Could you check a few things on this model? Use its own coordinates, in mm. A direction names the side the tool comes from. Round coordinates to 2 decimals unless told otherwise and drop trailing zeros. Loops run counter-clockwise (first coordinate to the right, second up) from the corner with the lowest first, then second, coordinate; pieces in that order, holes last. Notation, with made-up numbers: (-30.75, 71.25) -> (-7.75, 71.25) arc R25 cw to (-7.75, 102.25) -> close; hole circle Ø10 at (83.5, 41). An arc over 180 degrees is marked (long way). Put each result on its own line as item: value. Start each with the question number.
1. I need wall thicknesses on line 1 (X direction, y = 0.5, z = 0.6); line 2 (Z direction, x = -34, y = -3.5); line 3 (Y direction, x = -61.5, z = -0.9). Which ranges of each line are inside material? Lowest first, please. Write a range as [from, to].
2. Imagine slicing it at A-A, the plane y = -9. Please give me the cut outline in (x, z), and give its area (3 significant figures).
3. Imagine slicing it at D-D, the plane x = -38.5. Please give me the cut outline in (y, z).
4. Imagine slicing it at C-C, the plane y = -0.5. Please give me the cut outline in (x, z), and give its area (3 significant figures).
5. If we mould it in two halves opening along X, with no side actions, what happens to faces 1 (the flat face through (-43.491, -9, 2)), 2 (the flat face through (-72.441, 13, 2)), 3 (the flat face through (-40, 0, -1.5))? For each: pulls with the +X half, pulls with the -X half, needs draft (parallel to the pull), parting line crosses it, or undercut.
6. Which directions (+Z, -Z, +X, -X, +Y, -Y) give clear straight access to the entire face, cutting with the end or side of a thin tool? Please do faces 4 (the flat face through (-48, 9, 2)), 5 (the flat face through (-60, 20, -1.5)), 6 (the cylindrical face through (-38.1, 17.54, -0.74)), 7 (the flat face through (-55.991, -9, 2)).
7. I'm going to push flat-ended pins straight in: P1, Ø8, axis at x = -49.74, y = 10.11, coming from the -Z side; P2, Ø1.8, axis at x = -49.5, y = 8.5, coming from the +Z side; P3, Ø1.6, axis at x = -48.5, z = 2.5, coming from the -Y side; P4, Ø4, axis at x = -47, y = -6.5, coming from the -Z side. Where does each tip first touch, or does it pass through?
8. Imagine slicing it at B-B, the plane x = -45.5. Please give me the cut outline in (y, z).
```python
from build123d import *

# Parameters (mm, degrees)
SKETCH_1_W          = 45.4
SKETCH_1_H          = 61
EXTRUDE_1_DEPTH     = 4
SKETCH_2_W          = 12.5
SKETCH_2_H          = 18
CUT_EXTRUDE_1_DEPTH = 3.2
SKETCH_4_R          = 1.6
CUT_EXTRUDE_2_DEPTH = 10
SKETCH_5_R          = 3
CUT_EXTRUDE_3_DEPTH = 2
SKETCH_3_R          = 3.05
EXTRUDE_2_DEPTH     = 1.5


with BuildPart() as part:
    # 草图1 → 凸台-拉伸1 (new body)
    with BuildSketch(Plane.XY):
        with Locations((-49.741035857, 13.111663348)):
            Rectangle(SKETCH_1_W, SKETCH_1_H)
    extrude(amount=EXTRUDE_1_DEPTH)

    # 草图2 → 切除-拉伸1 (cut)
    with BuildSketch(Plane(origin=(0, 0, 0), x_dir=(-1, 0, 0), z_dir=(0, 0, -1))):
        with Locations((49.741035857, -8.388336652)):
            Rectangle(SKETCH_2_W, SKETCH_2_H)
    extrude(amount=-CUT_EXTRUDE_1_DEPTH, mode=Mode.SUBTRACT)

    # 草图4 → 切除-拉伸2 (cut)
    with BuildSketch(Plane.XY.offset(4)):
        with Locations((-49.741035857, 10.111663348)):
            Circle(SKETCH_4_R)
    extrude(amount=-CUT_EXTRUDE_2_DEPTH, mode=Mode.SUBTRACT)

    # 草图5 → 切除-拉伸3 (cut)
    with BuildSketch(Plane.XY.offset(4)):
        with Locations((-49.741035857, 10.111663348)):
            Circle(SKETCH_5_R)
    extrude(amount=-CUT_EXTRUDE_3_DEPTH, mode=Mode.SUBTRACT)

    # 草图3 → 凸台-拉伸2 (add)
    with BuildSketch(Plane(origin=(0, 0, 0), x_dir=(-1, 0, 0), z_dir=(0, 0, -1))):
        with Locations(Location((39.741035857, 0.111663348, 0), (0, 0, 180))):
            Circle(SKETCH_3_R)
        with Locations(Location((39.741035857, 20.111663348, 0), (0, 0, 180))):
            Circle(SKETCH_3_R)
        with Locations((59.741035857, 0.111663348)):
            Circle(SKETCH_3_R)
        with Locations((59.741035857, 20.111663348)):
            Circle(SKETCH_3_R)
    extrude(amount=EXTRUDE_2_DEPTH)


solid = part.part
```
Entries:
1. line 1: [-72.44, -55.99], [-43.49, -27.04]
1. line 2: [0, 4]
1. line 3: [-2.38, 2.6], [17.62, 22.6]
2. outline: (-72.44, 0) -> (-55.99, 0) -> (-55.99, 3.2) -> (-43.49, 3.2) -> (-43.49, 0) -> (-27.04, 0) -> (-27.04, 4) -> (-72.44, 4) -> close
2. area: 142 mm^2
3. outline: (-17.39, 0) -> (-2.67, 0) -> (-2.67, -1.5) -> (2.9, -1.5) -> (2.9, 0) -> (17.33, 0) -> (17.33, -1.5) -> (22.9, -1.5) -> (22.9, 0) -> (43.61, 0) -> (43.61, 4) -> (-17.39, 4) -> close
4. outline: (-72.44, 0) -> (-62.73, 0) -> (-62.73, -1.5) -> (-56.75, -1.5) -> (-56.75, 0) -> (-55.99, 0) -> (-55.99, 3.2) -> (-43.49, 3.2) -> (-43.49, 0) -> (-42.73, 0) -> (-42.73, -1.5) -> (-36.75, -1.5) -> (-36.75, 0) -> (-27.04, 0) -> (-27.04, 4) -> (-72.44, 4) -> close
4. area: 160 mm^2
5. face 1: undercut
5. face 2: pulls with the -X half
5. face 3: needs draft
6. face 4: +Z
6. face 5: -Z, +X, -X, +Y, -Y
6. face 6: -Z
6. face 7: -Z, -Y
7. P1: z = 0
7. P2: z = 2
7. P3: y = -17.39
7. P4: z = 3.2
8. outline: (-17.39, 3.2) -> (0.61, 3.2) -> (0.61, 0) -> (43.61, 0) -> (43.61, 4) -> (-17.39, 4) -> close
